Geometry: final body of the model. Coordinates: model frame, mm. Face numbers are marked on the shaded views. A direction names the side the tool comes from. Give positions to 0.01 mm unless a question says otherwise; leave off trailing zeros. Write each loop counter-clockwise with the first axis right and the second up, starting at its lowest first coordinate (ties: lowest second). Pieces come first, ordered by that corner, then holes. Notation, with made-up numbers: (-19, 35.5) -> (34, 35.5) arc R4 cw to (34, 40.5) -> close; hole circle Ø8 at (35.5, -39.5). An arc over 180 degrees is marked (long way). Answer in a Markdown table with one row per item. Add a question column.
from build123d import *

# Parameters (mm, degrees)
CROQUIS1_R                 = 8.5
SALIENTE_EXTRUIR1_DEPTH    = 30
CORTAR_EXTRUIR1_DEPTH      = 8.5
CROQUIS9_R                 = 11.15
SALIENTE_EXTRUIR5_DEPTH    = 20
CROQUIS3_R                 = 9.53
CORTAR_EXTRUIR2_DEPTH      = 19
CORTAR_EXTRUIR3_REACH      = 26.691
CROQUIS4_R                 = 2.035
CORTAR_EXTRUIR4_DEPTH      = 34.891665642
CORTAR_EXTRUIR4_DEPTH_BACK = 34.891665642
CROQUIS5_R                 = 2.025
CROQUIS7_R                 = 8.5
SALIENTE_EXTRUIR3_DEPTH    = 3
REDONDEO1_R                = 10


with BuildPart() as part:
    # Croquis1 → Saliente-Extruir1 (new body)
    with BuildSketch(Plane(origin=(0, 0, 0), x_dir=(0, 0, -1), z_dir=(1, 0, 0))):
        Circle(CROQUIS1_R)
    extrude(amount=SALIENTE_EXTRUIR1_DEPTH)

    # Croquis2 → Cortar-Extruir1 (cut)
    with BuildSketch(Plane(origin=(30, 0, 0), x_dir=(0, 0, -1), z_dir=(1, 0, 0))):
        Polygon((0, -6.962844246), (6.03, -3.481422123), (6.03, 3.481422123), (0, 6.962844246), (-6.03, 3.481422123), (-6.03, -3.481422123), align=None)
    extrude(amount=-CORTAR_EXTRUIR1_DEPTH, mode=Mode.SUBTRACT)

    # Croquis9 → Saliente-Extruir5 (add)
    with BuildSketch(Plane.ZY):
        Circle(CROQUIS9_R)
    extrude(amount=-SALIENTE_EXTRUIR5_DEPTH)

    # Croquis3 → Cortar-Extruir2 (cut)
    with BuildSketch(Plane.ZY):
        Circle(CROQUIS3_R)
    extrude(amount=-CORTAR_EXTRUIR2_DEPTH, mode=Mode.SUBTRACT)

    # Croquis4 → Cortar-Extruir3 (cut, up to next)
    with BuildSketch(Plane.ZY.offset(-19), mode=Mode.PRIVATE) as cortar_extruir3_sk1:
        Circle(CROQUIS4_R)
    cortar_extruir3_tool1 = extrude(cortar_extruir3_sk1.sketch, amount=-CORTAR_EXTRUIR3_REACH, mode=Mode.PRIVATE) & part.part
    add(cortar_extruir3_tool1.solids().sort_by_distance((19, 0, 0))[0], mode=Mode.SUBTRACT)

    # Croquis5 → Cortar-Extruir4 (cut, two sides: drawn at the far end of the back side and taken through both)
    with BuildSketch(Plane.XY.offset(-CORTAR_EXTRUIR4_DEPTH_BACK)):
        with Locations((6, 0)):
            Circle(CROQUIS5_R)
    extrude(amount=CORTAR_EXTRUIR4_DEPTH + CORTAR_EXTRUIR4_DEPTH_BACK, mode=Mode.SUBTRACT)

    # Croquis7 → Saliente-Extruir3 (add)
    with BuildSketch(Plane(origin=(30, 0, 0), x_dir=(0, 0, -1), z_dir=(1, 0, 0))):
        with Locations(Location((0, 0, 0), (0, 0, 180))):
            Circle(CROQUIS7_R)
        Polygon((-6.03, -3.481422123), (0, -6.962844246), (6.03, -3.481422123), (6.03, 3.481422123), (0, 6.962844246), (-6.03, 3.481422123), align=None, mode=Mode.SUBTRACT)
    extrude(amount=SALIENTE_EXTRUIR3_DEPTH)

    # Redondeo1
    # the kernel refuses this fillet: 10 mm, written as the material it adds along each edge
    with BuildSketch(Plane(origin=(20, 0, 0), x_dir=(0, 0, -1), z_dir=(0, 1, 0))) as redondeo1_piece_1:
        with BuildLine():
            CenterArc((18.5, -6.780671058), REDONDEO1_R, 137.307216105, 42.692783895)
            Line((11.15, 0), (11.003, 0.135613421))
            ThreePointArc((11.003, 0.135613421), (9.825, 0.2), (8.5, 0.2))
            Line((8.5, 0.2), (8.3, 0))
            Line((8.3, 0), (8.3, -6.780671058))
            Line((8.3, -6.780671058), (8.5, -6.780671058))
        make_face()
    revolve(axis=Axis((20, 0, 0), (-1, 0, 0)))


solid = part.part
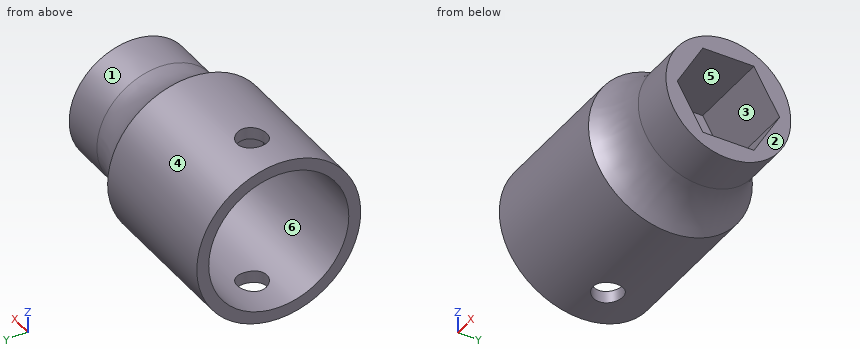
Q1. Section C-C on x = 2.5. Return loops of the section in (y, z), and give its area (3 significant figures).
Q2. Access query for the marked faces 4, 5 and 6. Directions: +Z, -Z, +X, -X, +Y, -Y. A direction counts if a zero-diameter tool reaches every point of the face in a straight line with its end or side. Return the directions, or none.
Q3. Section B-B on x = 6. Return loops of the section in (y, z) (3 decimals), and give its area (3 significant figures).
Q4. Pull-direction query (Z, two-part tool) for the marked faces 1, 2 and 3; classes: +Z half, -Z half, draft (parallel to the pull), parting line (faces both ways), or undercut.
Q5. Section D-D on y = -1. Count the separate pieces of the cut face and the enclosed holes in it, and give its area (3 significant figures).
Q6. Contact query for flat-ended pins moving along their axis: pin 1 Ø2 at (x, y) = (29.5, -1) entering from +Z; pin 2 Ø6 at (y, z) = (-5, -1) entering from -X; pin 3 Ø8 at (x, z) = (13, 6) entering from +Y. Output: stop coordinate, or through.
Q7. Line query: probe 1 along Z at (x, y) = (13, 0); probe 2 along Y at (x, z) = (31, 2.75). Output: solid intervals per line, ascending. Write a range as from..to.
Checks:
| question | item | result |
|---|---|---|
| 1 | outline | circle Ø22.3 at (0, 0); hole circle Ø19.06 at (0, 0) |
| 1 | area | 105 mm^2 |
| 2 | face 4 | +X, -X |
| 2 | face 5 | +X |
| 2 | face 6 | -X |
| 3 | outline | (-2.025, -10.965) -> (-2.025, -9.312) arc R9.53 cw to (-2.025, 9.312) -> (-2.025, 10.965) arc R11.15 ccw to start; (2.025, -10.965) arc R11.15 ccw to (2.025, 10.965) -> (2.025, 9.312) arc R9.53 cw to (2.025, -9.312) -> close |
| 3 | area | 92.0 mm^2 |
| 4 | face 1 | parting line |
| 4 | face 2 | draft |
| 4 | face 3 | undercut |
| 5 | separate pieces | 4 |
| 5 | enclosed holes | 0 |
| 5 | area | 156 mm^2 |
| 6 | pin 1 | z = 8.5 |
| 6 | pin 2 | x = 19 |
| 6 | pin 3 | y = 10.97 |
| 7 | probe 1 | -11.15..-9.53, 9.53..11.15 |
| 7 | probe 2 | -8.04..-5.38, 5.38..8.04 |
